```python
from build123d import *

# Parameters (mm, degrees)
EXTRUDE_1_DEPTH                 = 24
HOLE_WIZARD_5_0_5_1_D           = 5
HOLE_WIZARD_5_0_5_1_CSINK_D     = 5.05
HOLE_WIZARD_5_0_5_1_CSINK_ANGLE = 90


with BuildPart() as part:
    # 草图1 → 凸台-拉伸1 (new body)
    with BuildSketch(Plane(origin=(0, 0, 0), x_dir=(1, 0, 0), z_dir=(0, 1, 0))):
        with BuildLine():
            Line((-26, 0), (-24, 0))
            ThreePointArc((-24, 0), (0, 24), (24, 0))
            Line((24, 0), (26, 0))
            ThreePointArc((26, 0), (0, 26), (-26, 0))
        make_face()
    extrude(amount=EXTRUDE_1_DEPTH)

    # Ø5.0 (5) 直径孔1 (through all)
    with Locations(Plane.XY):
        with Locations((0, 12)):
            CounterSinkHole(HOLE_WIZARD_5_0_5_1_D / 2, HOLE_WIZARD_5_0_5_1_CSINK_D / 2, counter_sink_angle=HOLE_WIZARD_5_0_5_1_CSINK_ANGLE)


solid = part.part
```
For this review, take the finished solid that the model builds, in its own axes (mm). Give positions to 0.01 mm unless a question says otherwise; leave off trailing zeros. Write each loop counter-clockwise with the first axis right and the second up, starting at its lowest first coordinate (ties: lowest second). Pieces come first, ordered by that corner, then holes. Notation, with made-up numbers: M 67,-27 L 72,-27 A16 ccw 72,-9 Z; hole C 67,69 d3. An arc over 180 degrees is marked long. Answer as CSV lines item,"result".
1. Draft analysis for pull direction X (two halves, no side actions). For faces 1 (the cylindrical face through (0.572, 9.165, -25.994)), 2 (the flat face through (0, 0, -25)), 3 (the cylindrical face through (-0.528, 9.165, -23.994)), state which applies: +X half, -X half, draft (parallel to the pull), parting line (faces both ways), or undercut.
Findings:
face 1,"parting line"
face 2,"draft"
face 3,"undercut"
2. For pin 1 (5 mm diameter, centred on y = 7.5, z = -12.5, fed in from +X); pin 2 (8 mm diameter, centred on x = 4.5, y = 11, fed in from -Z); pin 3 (4 mm diameter, centred on x = 10.5, y = 21, fed in from +Z), all flat-tipped, find the tip position at first contact; note any pin that passes through.
Findings:
pin 1,"stops at x = 24"
pin 2,"stops at z = -25.99"
pin 3,"stops at z = -20.49"
3. Wall thickness on line 1 (Y direction, x = 0, z = -25.35); line 2 (X direction, y = 22, z = -18.75); line 3 (X direction, y = 17.25, z = -5): over which ranges is each line inside the solid? List them lowest first.
Findings:
line 1,"y = 0 to 9.5, 14.5 to 24"
line 2,"x = -18.01 to -14.98, 14.98 to 18.01"
line 3,"x = -25.51 to -23.47, 23.47 to 25.51"
4. Consider section C-C, the plane y = 22. Write out the cut boundary in (x, z).
Findings:
outline,"M -26,0 A26 ccw 26,0 L 24,0 A24 cw -24,0 Z"
5. Consider section A-A, the plane x = 0. Write out the cut boundary in (y, z), then the cut area to 3 significant figures.
Findings:
outline,"M 0,-26 L 9.5,-26 L 9.5,-24 L 0,-24 Z; M 14.5,-26 L 24,-26 L 24,-24 L 14.5,-24 Z"
area,"38.0 mm2"
6. Consider section D-D, the plane x = -17.5. Write out the cut boundary in (y, z), then the cut area to 3 significant figures.
Findings:
outline,"M 0,-19.23 L 24,-19.23 L 24,-16.42 L 0,-16.42 Z"
area,"67.3 mm2"
7. Consider section B-B, the plane z = -11.75. Write out the cut boundary in (x, y), then the cut area to 3 significant figures.
Findings:
outline,"M -23.19,0 L -20.93,0 L -20.93,24 L -23.19,24 Z; M 20.93,0 L 23.19,0 L 23.19,24 L 20.93,24 Z"
area,"109 mm2"
